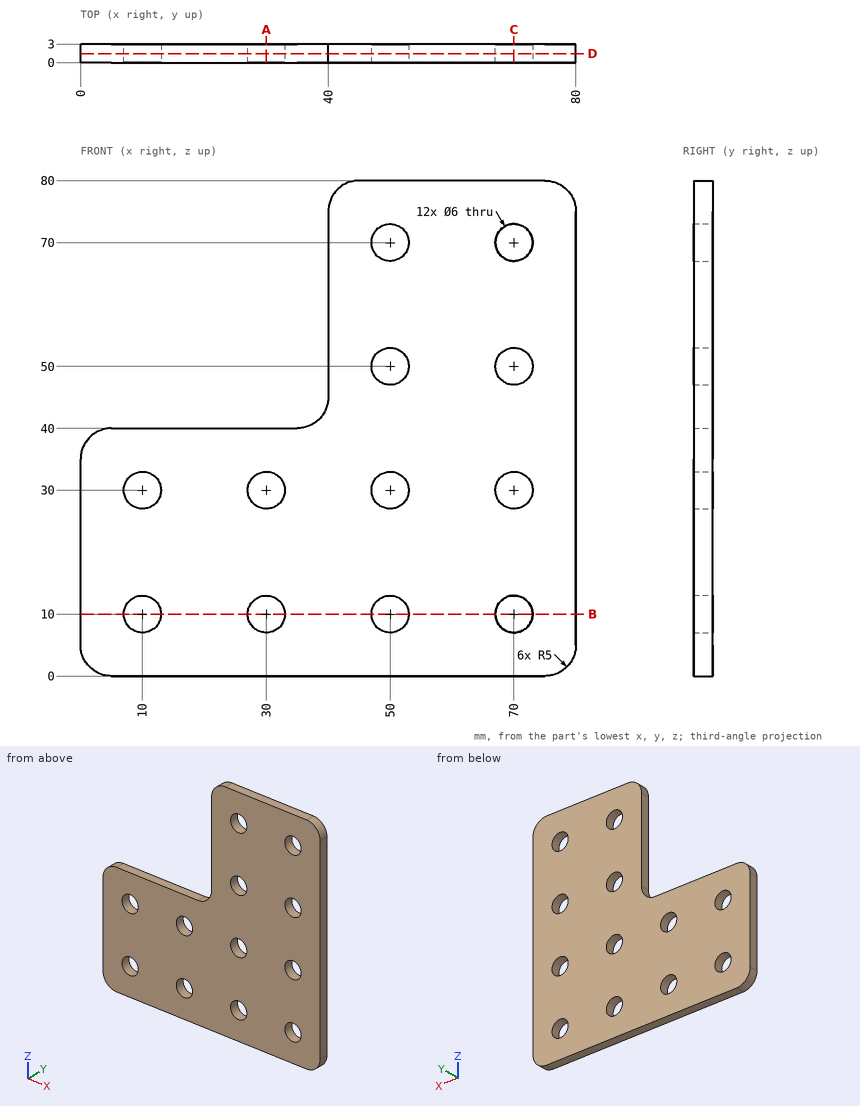
Geometry: see drawing. Coordinates: mm, zero at the bounding-box minimum. Give positions to 0.01 mm unless a question says otherwise; leave off trailing zeros. Order: outer loops, then holes, each group sorted by start corner. A loop starts at its lowest first (then second) coordinate and runs counter-clockwise, first axis right, second up.
Q1. Ray query, probe 1 along Z at (x, y) = (70, 2.1); probe 2 along X at (y, z) = (1.75, 50); probe 3 along Z at (x, y) = (30, 1.4). Return the intervals inside material, ascending.
Checked values:
probe 1: z = 0 to 7, 13 to 27, 33 to 47, 53 to 67, 73 to 80
probe 2: x = 40 to 47, 53 to 67, 73 to 80
probe 3: z = 0 to 7, 13 to 27, 33 to 40
Q2. Section B-B on z = 10. Output: boundary loops of the cut face in (x, y), and give its area (3 significant figures).
Checked values:
outline: (0, 0) - (7, 0) - (7, 3) - (0, 3) - close; (13, 0) - (27, 0) - (27, 3) - (13, 3) - close; (33, 0) - (47, 0) - (47, 3) - (33, 3) - close; (53, 0) - (67, 0) - (67, 3) - (53, 3) - close; (73, 0) - (80, 0) - (80, 3) - (73, 3) - close
area: 168 mm2
Q3. Section D-D on y = 1.45. State how many separate pieces and enclosed holes the cut face has, and give its area (3 significant figures).
Checked values:
separate pieces: 1
enclosed holes: 12
area: 4,440 mm2
Q4. Contact query for flat-ended pins moving along their axis: pin 1 Ø7 at (x, z) = (70, 10) entering from -Y; pin 2 Ø1.5 at (y, z) = (1.5, 56.5) entering from -X; pin 3 Ø5.5 at (x, z) = (70, 70) entering from +Y. Output: stop coordinate, or through.
Checked values:
pin 1: stops at y = 0
pin 2: stops at x = 40
pin 3: passes through
Q5. Section C-C on x = 70. Output: boundary loops of the cut face in (y, z).
Checked values:
outline: (0, 0) - (3, 0) - (3, 7) - (0, 7) - close; (0, 13) - (3, 13) - (3, 27) - (0, 27) - close; (0, 33) - (3, 33) - (3, 47) - (0, 47) - close; (0, 53) - (3, 53) - (3, 67) - (0, 67) - close; (0, 73) - (3, 73) - (3, 80) - (0, 80) - close
Q6. Section A-A on x = 30. Output: boundary loops of the cut face in (y, z).
Checked values:
outline: (0, 0) - (3, 0) - (3, 7) - (0, 7) - close; (0, 13) - (3, 13) - (3, 27) - (0, 27) - close; (0, 33) - (3, 33) - (3, 40) - (0, 40) - close
